```python
from build123d import *

# Parameters (mm, degrees)
F0_W     = 101.6
F0_H     = 76.2
F1_DEPTH = 7.9375
F2_R     = 3.9624
F2_W     = 12.7
F2_H     = 50.8
F3_DEPTH = 25.4


with BuildPart() as f1:
    # F0 (on Front) → F1 (new body, symmetric)
    with BuildSketch(Plane.XZ):
        Rectangle(F0_W, F0_H)
    extrude(amount=F1_DEPTH, both=True)

    # F2 (on Front) → F3 (join)
    with BuildSketch(Plane.XZ):
        with Locations((34.163, 21.463)):
            Circle(F2_R)
        with Locations((34.163, -21.463)):
            Circle(F2_R)
        Rectangle(F2_W, F2_H)
        with Locations((-34.163, 21.463)):
            Circle(F2_R)
        with Locations((-34.163, -21.463)):
            Circle(F2_R)
    extrude(amount=F3_DEPTH)


solid = f1.part
```
Here's how the part is built. I have some questions about the finished solid (model axes, mm). A direction names the side the tool comes from. Give positions to 0.01 mm unless a question says otherwise; leave off trailing zeros. Write each loop counter-clockwise with the first axis right and the second up, starting at its lowest first coordinate (ties: lowest second). Pieces come first, ordered by that corner, then holes. Notation, with made-up numbers: M -0.5,0 L 30.5,0 A13 cw 30.5,12 Z; hole C 22.5,18 d10. An arc over 180 degrees is marked long. Put each result on its own line as item: value. Start each with the question number.
Item 1: On a 3-axis mill with a long thin cutter (end or side, diameter ignored), from which of +Z, -Z, +X, -X, +Y, -Y can I reach the whole of each face in a straight line? I mean faces 4 (the flat face through (-1, 0, 38.1)), 5 (the cylindrical face through (30.204, -16.547, 21.637)), 6 (the flat face through (6.35, -17, 0)). Say none if no direction works.
Item 2: Will these pins go through, and if not, where does the flat tip stop? pin 1 (2 mm diameter, centred on x = 16.5, z = 22.5, fed in from -Y); pin 2 (14 mm diameter, centred on y = -19.5, z = -3, fed in from -X); pin 3 (6.5 mm diameter, centred on x = -2, y = -13, fed in from +Z).
Item 3: If we section it at B-B, the plane z = -8: Write out the boundary of the cut face in (x, y), then the cut area to 3 significant figures.
Item 4: If we section it at D-D, the plane z = 23.5: Write out the boundary of the cut face in (x, y), then the cut area to 3 significant figures.
Item 5: If we section it at C-C, the plane x = 3: Write out the boundary of the cut face in (y, z).
Item 6: I need wall thicknesses on L1, parallel to Y at x = 16.5, z = -6.5; L2, parallel to X at y = -15.5, z = 2. Which ranges of each line are inside material? Lowest first, please. Write a range as from..to.
Item 7: If we section it at A-A, the plane y = -11: Write out the boundary of the cut face in (x, z).
Item 8: Thinking about a two-plate mould opening in X: for faces 1 (the flat face through (34, -25.4, 22)), 2 (the cylindrical face through (-32.335, -16.547, -24.978)), 3 (the flat face through (50.8, 0, -1)), which applies, +X half, -X half, draft (parallel to the pull), parting line (faces both ways), or undercut?
Values:
1. face 4: +Z, +X, -X, +Y, -Y
1. face 5: -Y
1. face 6: +Z, -Z, -Y
2. pin 1: y = -7.94
2. pin 2: x = -6.35
2. pin 3: z = 25.4
3. outline: M -50.8,-7.94 L -6.35,-7.94 L -6.35,-25.4 L 6.35,-25.4 L 6.35,-7.94 L 50.8,-7.94 L 50.8,7.94 L -50.8,7.94 Z
3. area: 1,830 mm²
4. outline: M -50.8,-7.94 L -37.56,-7.94 L -37.56,-25.4 L -30.76,-25.4 L -30.76,-7.94 L -6.35,-7.94 L -6.35,-25.4 L 6.35,-25.4 L 6.35,-7.94 L 30.76,-7.94 L 30.76,-25.4 L 37.56,-25.4 L 37.56,-7.94 L 50.8,-7.94 L 50.8,7.94 L -50.8,7.94 Z
4. area: 2,070 mm²
5. outline: M -25.4,-25.4 L -7.94,-25.4 L -7.94,-38.1 L 7.94,-38.1 L 7.94,38.1 L -7.94,38.1 L -7.94,25.4 L -25.4,25.4 Z
6. L1: -7.94..7.94
6. L2: -6.35..6.35
7. outline: C -34.16,-21.46 d7.92; C -34.16,21.46 d7.92; M -6.35,-25.4 L 6.35,-25.4 L 6.35,25.4 L -6.35,25.4 Z; C 34.16,-21.46 d7.92; C 34.16,21.46 d7.92
8. face 1: draft
8. face 2: undercut
8. face 3: +X half
